Part model, mm, in its own coordinate system. A direction names the side the tool comes from. Coordinates: 2 decimals unless noted, no trailing zeros. Loops run counter-clockwise (first coordinate to the right, second up) from the corner with the lowest first, then second, coordinate; pieces in that order, holes last. Notation, with made-up numbers: (7.25, 41.25) -> (22.25, 41.25) arc R12 ccw to (22.25, 53.25) -> close; hole circle Ø11 at (61, -6.5). An arc over 180 degrees is marked (long way). Use one line per item in the form item = value. Start each with the question number.
(1) Band-saw the part on C-C on z = 2.45. Give the cut face in (x, y), then the cut area to 3 significant figures.
(2) Drill centre lines: L1, parallel to Y at x = -3, z = 0.3; L2, parallel to Y at x = 83, z = 0.3; L3, parallel to X at y = 111, z = 4.95. Where is each one in solid material? Low to high. Write a range as [from, to].
(3) 3-axis set-ups, long thin cutter, end or side, ignore diameter. For faces 3 (the flat face through (233, 17, 0.5)), 4 (the flat face through (-3, 143.4, 0.5)), 5 (the flat face through (166, 152, 0.5)), 6 (the flat face through (147, -3, 0.5)): which of +Z, -Z, +X, -X, +Y, -Y reach the whole face in a straight line?
(4) Mould opens along Y. For faces 1 (the flat face through (113, 76, 0)), 2 (the flat face through (112, 77, 4.7)) say: +Y half, -Y half, draft (parallel to the pull), parting line (faces both ways), or undercut.
(5) Band-saw the part on A-A on y = 104.5. Give the cut face in (x, z), then the cut area to 3 significant figures.
(6) Pin check, flat tips, straight feed: P1, Ø3.5, axis at x = 167.96, y = 152.2, coming from the -Z side; P2, Ø1, axis at y = 76, z = 4.5, coming from the +X side; P3, Ø5.5, axis at x = 82.5, y = 153.5, coming from the +Z side; P4, Ø8, axis at x = 49.5, y = 16, coming from the +Z side. Stop position of each tip, or through.
(7) Band-saw the part on B-B on x = 199. Give the cut face in (y, z), then the cut area to 3 significant figures.
```python
from build123d import *

# Parameters (mm, degrees)
SKETCH1_W                  = 229.46
SKETCH1_H                  = 149.2
BOSS_EXTRUDE1_DEPTH        = 5.2
SKETCH2_W                  = 220.76
SKETCH2_H                  = 139
CUT_EXTRUDE1_DEPTH         = 0.5
SKETCH3_W                  = 6
SKETCH3_H                  = 5
SKETCH3_H_2                = 11
SKETCH3_W_2                = 5
SKETCH3_H_3                = 6
BOSS_EXTRUDE2_DEPTH        = 0.5
SKETCH4_W                  = 5
SKETCH4_H                  = 6
BOSS_EXTRUDE3_DEPTH        = 0.5
F_3_1_3_1_DIAMETER_HOLE1_D = 3.1
F_3_1_3_1_DIAMETER_HOLE4_D = 3.1
F_2_5_2_5_DIAMETER_HOLE2_D = 2.5
F_3_0_3_DIAMETER_HOLE1_D   = 3


with BuildPart() as part:
    # Sketch1 → Boss-Extrude1 (new body)
    with BuildSketch(Plane.XY):
        with Locations((114.73, 74.6)):
            Rectangle(SKETCH1_W, SKETCH1_H)
    extrude(amount=BOSS_EXTRUDE1_DEPTH)

    # Sketch2 → Cut-Extrude1 (cut)
    with BuildSketch(Plane.XY.offset(5.2)):
        with Locations((113.98, 75.9)):
            Rectangle(SKETCH2_W, SKETCH2_H)
    extrude(amount=-CUT_EXTRUDE1_DEPTH, mode=Mode.SUBTRACT)

    # Sketch3 → Boss-Extrude2 (add)
    with BuildSketch(Plane(origin=(0, 0, 0), x_dir=(-1, 0, 0), z_dir=(0, 0, -1))):
        with Locations((-232.46, 141.7)):
            Rectangle(SKETCH3_W, SKETCH3_H)
        with Locations((-232.46, 16.5)):
            Rectangle(SKETCH3_W, SKETCH3_H_2)
        with Locations((-148.96, -3)):
            Rectangle(SKETCH3_W_2, SKETCH3_H_3)
        with Locations((-88.5, -3)):
            Rectangle(SKETCH3_W_2, SKETCH3_H_3)
        with Locations((3, 21.5)):
            Rectangle(SKETCH3_W, SKETCH3_H_2)
        with Locations((3, 141.7)):
            Rectangle(SKETCH3_W, SKETCH3_H)
    extrude(amount=-BOSS_EXTRUDE2_DEPTH)

    # Sketch4 → Boss-Extrude3 (add)
    with BuildSketch(Plane(origin=(0, 0, 0), x_dir=(-1, 0, 0), z_dir=(0, 0, -1))):
        with Locations((-167.96, 152.2)):
            Rectangle(SKETCH4_W, SKETCH4_H)
        with Locations((-83, 152.2)):
            Rectangle(SKETCH4_W, SKETCH4_H)
    extrude(amount=-BOSS_EXTRUDE3_DEPTH)

    # Ø3.1 (3.1) Diameter Hole1 (through all)
    with Locations(Plane.XY.offset(0.5)):
        with Locations((-3, 141.7), (83, 152.2), (167.96, 152.2), (232.46, 141.7), (148.96, -3), (88.5, -3)):
            Hole(F_3_1_3_1_DIAMETER_HOLE1_D / 2)

    # Ø3.1 (3.1) Diameter Hole4 (through all)
    with Locations(Plane.XY.offset(0.5)):
        with Locations((232.618638534, 14)):
            Hole(F_3_1_3_1_DIAMETER_HOLE4_D / 2)

    # Ø2.5 (2.5) Diameter Hole2 (through all)
    with Locations(Plane.XY.offset(0.5)):
        with Locations((-3, 24), (-2.932911523, 19)):
            Hole(F_2_5_2_5_DIAMETER_HOLE2_D / 2)

    # Ø3.0 (3) Diameter Hole1 (through all)
    with Locations(Plane.XY.offset(0.5)):
        with Locations((232.618638534, 19)):
            Hole(F_3_0_3_DIAMETER_HOLE1_D / 2)


solid = part.part
```
A:
q1.outline = (0, 0) -> (229.46, 0) -> (229.46, 149.2) -> (0, 149.2) -> close
q1.area = 34,200 mm²
q2.L1 = [16, 17.75], [20.25, 22.75], [25.25, 27], [139.2, 140.15], [143.25, 144.2]
q2.L2 = [0, 150.65], [153.75, 155.2]
q2.L3 = [0, 3.6], [224.36, 229.46]
q3.face_3 = +Z, +X, +Y, -Y
q3.face_4 = +Z, -X, +Y, -Y
q3.face_5 = +Z, +X, -X, +Y
q3.face_6 = +Z, +X, -X, -Y
q4.face_1 = draft
q4.face_2 = undercut
q5.outline = (0, 0) -> (229.46, 0) -> (229.46, 5.2) -> (224.36, 5.2) -> (224.36, 4.7) -> (3.6, 4.7) -> (3.6, 5.2) -> (0, 5.2) -> close
q5.area = 1,080 mm²
q6.P1 = 0
q6.P2 = 229.46
q6.P3 = 0.5
q6.P4 = 4.7
q7.outline = (0, 0) -> (149.2, 0) -> (149.2, 5.2) -> (145.4, 5.2) -> (145.4, 4.7) -> (6.4, 4.7) -> (6.4, 5.2) -> (0, 5.2) -> close
q7.area = 706 mm²
